Can you work these out from the model? Positions are in its coordinate system, mm. A direction names the side the tool comes from. Coordinates: 2 decimals unless noted, no trailing zeros. Order: outer loops, then holes, each group sorted by start corner. A loop starts at its lowest first (then second) coordinate and runs counter-clockwise, first axis right, second up. Notation, with made-up numbers: M 3.5,-7 L 14.5,-7 A33 cw 14.5,27 Z; hole C 0,5 d4. An arc over 180 degrees is marked long. Answer as a JSON object with one key per item and string values.
Autodesk Inventor part; units mm, degrees
ref_plane "YZ Plane" through (0, 0, 0) normal (1, 0, 0) x (0, 1, 0)
ref_plane "XZ Plane" through (0, 0, 0) normal (0, 1, 0) x (-1, 0, 0)
ref_plane "XY Plane" through (0, 0, 0) normal (0, 0, 1) x (1, 0, 0)
sketch "Sketch1" plane through (0, 0, 0) normal (0, 0, 1) x (1, 0, 0)
  line L0 (0, 0) -> (252.4125, 0)
  line L1 (252.4125, 0) -> (252.4125, 244.475)
  line L2 (252.4125, 244.475) -> (0, 244.475)
  line L3 (0, 244.475) -> (0, 0)
  dimension "d0" = 252.4125
  dimension "d1" = 244.475
extrude "Extrusion1" add sketch "Sketch1" along normal blind 19.05
sketch "Sketch3" plane through (0, 0, 19.05) normal (0, 0, 1) x (1, 0, 0)
  line L0 (0, 0) -> (252.4125, 0)
  line L1 (252.4125, 244.475) -> (0, 244.475)
  line L2 (0, 244.475) -> (0, 0)
  line L3 (0, 244.475) -> (19.05, 244.475)
  line L4 (19.05, 244.475) -> (19.05, 225.425)
  line L5 (19.05, 225.425) -> (0, 225.425)
  line L6 (0, 225.425) -> (0, 244.475)
  line L7 (19.05, 168.275) -> (0, 168.275)
  line L8 (0, 168.275) -> (0, 149.225)
  line L9 (0, 149.225) -> (19.05, 149.225)
  line L10 (19.05, 149.225) -> (19.05, 168.275)
  line L11 (0, 130.175) -> (19.05, 130.175)
  line L12 (19.05, 130.175) -> (19.05, 111.125)
  line L13 (19.05, 111.125) -> (0, 111.125)
  line L14 (0, 111.125) -> (0, 130.175)
  line L15 (0, 206.375) -> (19.05, 206.375)
  line L16 (19.05, 206.375) -> (19.05, 187.325)
  line L17 (19.05, 187.325) -> (0, 187.325)
  line L18 (0, 187.325) -> (0, 206.375)
  line L19 (0, 92.075) -> (19.05, 92.075)
  line L20 (19.05, 92.075) -> (19.05, 73.025)
  line L21 (19.05, 73.025) -> (0, 73.025)
  line L22 (0, 73.025) -> (0, 92.075)
  line L23 (0, 53.975) -> (19.05, 53.975)
  line L24 (19.05, 53.975) -> (19.05, 34.925)
  line L25 (19.05, 34.925) -> (0, 34.925)
  line L26 (0, 34.925) -> (0, 53.975)
  line L27 (0, 15.875) -> (19.05, 15.875)
  line L28 (19.05, 15.875) -> (19.05, -3.175)
  line L29 (19.05, -3.175) -> (0, -3.175)
  line L30 (0, -3.175) -> (0, 15.875)
  dimension "d4" = 19.05
  dimension "d5" = 19.05
  dimension "d6" = 244.475
  dimension "d7" = 19.05
  dimension "d8" = 19.05
  dimension "d9" = 19.05
  dimension "d10" = 19.05
  dimension "d11" = 19.05
  dimension "d12" = 19.05
  dimension "d13" = 19.05
  dimension "d14" = 19.05
  dimension "d15" = 19.05
  dimension "d16" = 19.05
  dimension "d17" = 19.05
  dimension "d18" = 19.05
  dimension "d19" = 19.05
  dimension "d20" = 19.05
  dimension "d21" = 19.05
  dimension "d22" = 19.05
  dimension "d23" = 19.05
  dimension "d24" = 15.875
extrude "Extrusion2" cut sketch "Sketch3" against normal through all
mirror "Mirror1" about plane through (252.4125, 0, 0) normal (1, 0, 0)
sketch "Sketch7" plane through (0, 0, 19.05) normal (0, 0, 1) x (1, 0, 0)
  line L0 (19.05, 34.925) -> (0, 34.925)
  line L1 (0, 34.925) -> (0, 15.875)
  line L2 (0, 15.875) -> (19.05, 15.875)
  line L3 (19.05, 15.875) -> (19.05, 0)
  line L4 (19.05, 0) -> (485.775, 0)
  line L5 (485.775, 15.875) -> (485.775, 0)
  line L6 (504.825, 15.875) -> (485.775, 15.875)
  line L7 (504.825, 34.925) -> (504.825, 15.875)
  line L8 (485.775, 34.925) -> (504.825, 34.925)
  line L9 (485.775, 53.975) -> (485.775, 34.925)
  line L10 (504.825, 53.975) -> (485.775, 53.975)
  line L11 (504.825, 73.025) -> (504.825, 53.975)
  line L12 (485.775, 73.025) -> (504.825, 73.025)
  line L13 (485.775, 92.075) -> (485.775, 73.025)
  line L14 (504.825, 92.075) -> (485.775, 92.075)
  line L15 (504.825, 111.125) -> (504.825, 92.075)
  line L16 (19.05, 244.475) -> (485.775, 244.475)
  line L17 (0, 111.125) -> (0, 92.075)
  line L18 (0, 92.075) -> (19.05, 92.075)
  line L19 (19.05, 92.075) -> (19.05, 73.025)
  line L20 (19.05, 73.025) -> (0, 73.025)
  line L21 (0, 73.025) -> (0, 53.975)
  line L22 (0, 53.975) -> (19.05, 53.975)
  line L23 (19.05, 53.975) -> (19.05, 34.925)
  line L24 (0, 100.0125) -> (504.825, 100.0125)
  point P0 (0, 0)
  dimension "d56" = 144.4625
extrude "Extrusion4" cut sketch "Sketch7" against normal through all
properties part number "deep_side" material "Wood (Birch)"
Item 1: I want a section at B-B, the plane y = 235.5. Write out the boundary of the cut face in (x, z) (3 decimals).
Answers follow:
{"outline": "M 19.05,0 L 485.775,0 L 485.775,19.05 L 19.05,19.05 Z"}
Item 2: Which directions (+Z, -Z, +X, -X, +Y, -Y) give clear straight access to the entire face, cutting with the end or side of a thin tool? Please do faces 5 (the flat face through (9, 149.225, 10)), 6 (the flat face through (495, 168.275, 10)), 7 (the flat face through (485.775, 235, 10)).
Answers follow:
{"face 5": "+Z, -Z, -X", "face 6": "+Z, -Z, +X", "face 7": "+Z, -Z, +X, +Y"}
Item 3: I'm going to push flat-ended pins straight in: pin 1 (9.5 mm diameter, centred on x = 7, z = 10.5, fed in from +Y) (3 decimals); pin 2 (9.5 mm diameter, centred on y = 195, z = 7.5, fed in from -X); pin 3 (5.5 mm diameter, centred on y = 231, z = 9.5, fed in from +X) (3 decimals). Where does each tip first touch, or does it pass through?
Answers follow:
{"pin 1": "stops at y = 225.425", "pin 2": "stops at x = 19.05", "pin 3": "stops at x = 485.775"}
Item 4: Please list where this line runs through material, in increasing order: line 1 (X direction, y = 232, z = 11.5) (3 decimals).
Answers follow:
{"line 1": "x = 19.05 to 485.775"}
Item 5: If we mould it in two halves opening along Y, with no side actions, what happens to faces 1 (the flat face through (9, 206.375, 10)), 2 (the flat face through (10, 225.425, 10)), 3 (the flat face through (0, 106, 9)), 4 (the flat face through (9, 130.175, 10))? For each: pulls with the +Y half, pulls with the -Y half, needs draft (parallel to the pull), parting line crosses it, or undercut.
Answers follow:
{"face 1": "undercut", "face 2": "pulls with the +Y half", "face 3": "needs draft", "face 4": "undercut"}
